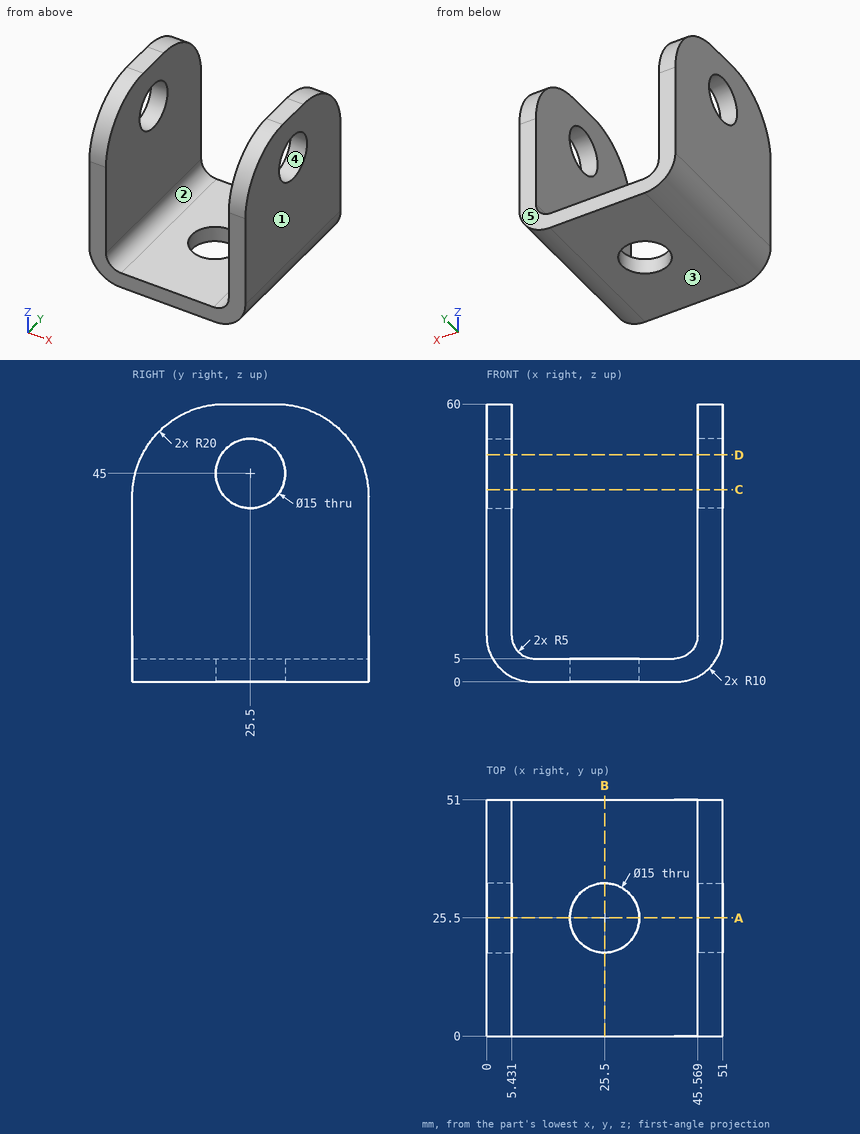
Answer from the drawing. Dimensions are ordinates in mm from the lowest x, y and z of the part. A direction names the side the tool comes from. Give positions to 0.01 mm unless a question says otherwise; leave off trailing zeros. Order: outer loops, then holes, each group sorted by start corner. A loop starts at its lowest first (then second) coordinate and runs counter-clockwise, first axis right, second up.
Item 1: The part is cut by section D-D, the plane z = 49. Give the vertices of the cut face in (x, y).
From the geometry:
outline: (0, 2.14) - (5.43, 2.14) - (5.43, 19.16) - (0, 19.16) - close; (0, 31.84) - (5.43, 31.84) - (5.43, 48.86) - (0, 48.86) - close; (45.57, 2.14) - (51, 2.14) - (51, 19.16) - (45.57, 19.16) - close; (45.57, 31.84) - (51, 31.84) - (51, 48.86) - (45.57, 48.86) - close
Item 2: The part is cut by section A-A, the plane y = 25.5. Give the vertices of the cut face in (x, z), and give its area (3 significant figures).
From the geometry:
outline: (0, 10) arc R10 ccw to (10, 0) - (18, 0) - (18, 5) - (10.43, 5) arc R5 cw to (5.43, 10) - (5.43, 37.5) - (0, 37.5) - close; (0, 52.5) - (5.43, 52.5) - (5.43, 60) - (0, 60) - close; (33, 0) - (41, 0) arc R10 ccw to (51, 10) - (51, 37.5) - (45.57, 37.5) - (45.57, 10) arc R5 cw to (40.57, 5) - (33, 5) - close; (45.57, 52.5) - (51, 52.5) - (51, 60) - (45.57, 60) - close
area: 582 mm2
Item 3: For a pull along Y with two mould halves and no side action, classify the marked faces 3, 4 and 5 as pulls with the +Y half, pulls with the -Y half, needs draft (parallel to the pull), parting line crosses it, or undercut.
From the geometry:
face 3: needs draft
face 4: undercut
face 5: pulls with the +Y half
Item 4: Which of the six approach directions +Z, -Z, +X, -X, +Y, -Y give full straight-line access (tool end or side, diameter ignored) to the marked faces 1 and 2?
From the geometry:
face 1: +Z, -Z, +X, +Y, -Y
face 2: +Z, +Y, -Y
Item 5: Find the intervals of material crossed by probe 1 along X at (y, z) = (34.5, 40); probe 2 along Y at (x, z) = (25.5, 1.15); probe 3 along Z at (x, y) = (36, 26.5), in increasing order.
From the geometry:
probe 1: x = 0 to 5.43, 45.57 to 51
probe 2: y = 0 to 18, 33 to 51
probe 3: z = 0 to 5
Item 6: The part is cut by section C-C, the plane z = 41.5. Give the vertices of the cut face in (x, y).
From the geometry:
outline: (0, 0.06) - (5.43, 0.06) - (5.43, 18.87) - (0, 18.87) - close; (0, 32.13) - (5.43, 32.13) - (5.43, 50.94) - (0, 50.94) - close; (45.57, 0.06) - (51, 0.06) - (51, 18.87) - (45.57, 18.87) - close; (45.57, 32.13) - (51, 32.13) - (51, 50.94) - (45.57, 50.94) - close
Item 7: Given pin 1 Ø2 at (x, y) = (42, 10) entering from +Z; pin 2 Ø8 at (x, y) = (33.5, 19) entering from +Z; pin 3 Ø5 at (x, z) = (42.5, 8.5) entering from -Y; pin 4 Ø19.5 at (y, z) = (25.5, 45) entering from +X, each flat-ended and moving along its own axis, determine where each tip first touches the part or whether it passes through.
From the geometry:
pin 1: stops at z = 5.63
pin 2: stops at z = 5
pin 3: passes through
pin 4: stops at x = 51
Item 8: The part is cut by section B-B, the plane x = 25.5. Give the vertices of the cut face in (y, z).
From the geometry:
outline: (0, 0) - (18, 0) - (18, 5) - (0, 5) - close; (33, 0) - (51, 0) - (51, 5) - (33, 5) - close
